CAD build for the part. Positions are in the model's coordinates, mm. A direction names the side the tool comes from. Coordinates: 2 decimals unless noted, no trailing zeros. Loops run counter-clockwise (first coordinate to the right, second up) from the corner with the lowest first, then second, coordinate; pieces in that order, holes last. Notation, with made-up numbers: (-6, 11.5) -> (53, 11.5) arc R25 cw to (53, 29.5) -> close; hole circle Ø1 at (3.25, 64). An arc over 180 degrees is marked (long way). Answer as CSV lines item,"result". Start each with the question number.
```python
from build123d import *

# Parameters (mm, degrees)
SKETCH1_W           = 152.4
SKETCH1_H           = 292.1
BOSS_EXTRUDE1_DEPTH = 3.048
SKETCH2_R           = 25.4
SKETCH2_R_2         = 10.7315
SKETCH2_R_3         = 2.0193
SKETCH2_W           = 16.173788568
SKETCH2_H           = 32.6898
CUT_EXTRUDE1_DEPTH  = 165.761442103
SKETCH4_W           = 55.88
SKETCH4_H           = 76.2
CUT_EXTRUDE2_DEPTH  = 165.761442103
SKETCH5_R           = 2.54
CUT_EXTRUDE3_DEPTH  = 165.761442103
SKETCH6_W           = 152.4
SKETCH6_H           = 5.08
CUT_EXTRUDE4_DEPTH  = 165.761442103
CUT_EXTRUDE5_DEPTH  = 6.35
FILLET1_R           = 6.35


with BuildPart() as part:
    # Sketch1 → Boss-Extrude1 (new body)
    with BuildSketch(Plane.XY):
        Rectangle(SKETCH1_W, SKETCH1_H)
    extrude(amount=BOSS_EXTRUDE1_DEPTH)

    # Sketch2 → Cut-Extrude1 (cut, through all)
    with BuildSketch(Plane.XY):
        with Locations(Location((0, -59.69, 0), (0, 0, 180))):
            Circle(SKETCH2_R)
        with Locations((0, 92.71)):
            Circle(SKETCH2_R_2)
        with Locations(Location((0, 38.1, 0), (0, 0, 180))):
            Circle(SKETCH2_R_3)
        with Locations(Location((0, 31.75, 0), (0, 0, 180))):
            Circle(SKETCH2_R_3)
        with Locations(Location((0, 25.4, 0), (0, 0, 180))):
            Circle(SKETCH2_R_3)
        with Locations(Location((0, 19.05, 0), (0, 0, 180))):
            Circle(SKETCH2_R_3)
        with Locations(Location((0, 12.7, 0), (0, 0, 180))):
            Circle(SKETCH2_R_3)
        with Locations(Location((0, 6.35, 0), (0, 0, 180))):
            Circle(SKETCH2_R_3)
        with Locations(Location((0, 0, 0), (0, 0, 180))):
            Circle(SKETCH2_R_3)
        with Locations(Location((0, -6.35, 0), (0, 0, 180))):
            Circle(SKETCH2_R_3)
        with Locations((0, 92.71)):
            Rectangle(SKETCH2_W, SKETCH2_H)
    extrude(amount=CUT_EXTRUDE1_DEPTH, mode=Mode.SUBTRACT)

    # Sketch4 → Cut-Extrude2 (cut, through all)
    with BuildSketch(Plane.XY):
        with Locations((48.26, 107.95)):
            Rectangle(SKETCH4_W, SKETCH4_H)
    extrude(amount=CUT_EXTRUDE2_DEPTH, mode=Mode.SUBTRACT)

    # Sketch5 → Cut-Extrude3 (cut, through all)
    with BuildSketch(Plane(origin=(0, 0, 0), x_dir=(-1, 0, 0), z_dir=(0, 0, -1))):
        with Locations((-38.1, -106.299)):
            Circle(SKETCH5_R)
        with Locations((-63.5, -106.299)):
            Circle(SKETCH5_R)
        with Locations((63.5, -106.299)):
            Circle(SKETCH5_R)
        with Locations((38.1, -106.299)):
            Circle(SKETCH5_R)
    extrude(amount=-CUT_EXTRUDE3_DEPTH, mode=Mode.SUBTRACT)

    # Sketch6 → Cut-Extrude4 (cut, through all)
    with BuildSketch(Plane(origin=(0, 0, 0), x_dir=(-1, 0, 0), z_dir=(0, 0, -1))):
        with Locations((0, -143.51)):
            Rectangle(SKETCH6_W, SKETCH6_H)
    extrude(amount=-CUT_EXTRUDE4_DEPTH, mode=Mode.SUBTRACT)

    # Sketch7 → Cut-Extrude5 (cut)
    with BuildSketch(Plane(origin=(0, 0, 0), x_dir=(-1, 0, 0), z_dir=(0, 0, -1))):
        with BuildLine():
            Line((63.5, 133.35), (15.671209909, 133.35))
            Line((15.671209909, 133.35), (15.671209909, -24.962155552))
            ThreePointArc((15.671209909, -24.962155552), (32.005336255, -39.019527068), (38.1, -59.69))
            Line((38.1, -59.69), (63.5, -59.69))
            Line((63.5, -59.69), (63.5, 133.35))
        make_face()
    extrude(amount=-CUT_EXTRUDE5_DEPTH, mode=Mode.SUBTRACT)

    # Fillet1
    fillet1_edges = [part.edges().sort_by_distance(p)[0] for p in [
        (-38.1, -59.69, 1.524),
        (-15.671209909, -24.962155552, 1.524),
        (-15.671209909, 133.35, 1.524),
        (-63.5, 133.35, 1.524),
        (-63.5, -59.69, 1.524),
    ]]
    fillet(fillet1_edges, radius=FILLET1_R)


solid = part.part
```
Q1. Saw through at A-A (x = 28). List the corners of the cut face in (y, z), and give its area (3 significant figures).
Q2. Saw through at B-B (z = 2.35). Give the number of separate pieces and of enclosed holes in the cut face, and give its area (3 significant figures).
Q3. Pin check, flat tips, straight feed: pin 1 Ø3.5 at (x, y) = (0, 19.05) entering from -Z; pin 2 Ø8 at (x, y) = (-38.1, -106.299) entering from -Z; pin 3 Ø1.5 at (x, z) = (60.5, 1.5) entering from +Y; pin 4 Ø1.5 at (y, z) = (105, 2) entering from +X. Stop position of each tip, or through.
Q4. Two-plate mould, pull along X, no slides. Class faces 1 (the flat face through (-1, -27, 0)), 2 (the cylindrical face through (-64.87, -104.16, 1.5)): pulls with the +X half, pulls with the -X half, needs draft (parallel to the pull), parting line crosses it, or undercut.
Q5. Probe probe 1 along X at (y, z) = (25.4, 1.55); probe 2 along Y at (x, z) = (63.5, 1.5); probe 3 along X at (y, z) = (-56.5, 1.1). List the from-to ranges inside material, lowest first. Write a range as from..to.
Q6. Which spindle directions (+Z, -Z, +X, -X, +Y, -Y) get a long thin tool onto all of the face, cutting with end or side? Do faces 3 (the cylindrical face through (-61.69, 131.44, 1.55)), 4 (the flat face through (-1, -27, 3.048)). Say none if no direction does.
Ans:
1,outline,"(-140.97, 0) -> (69.85, 0) -> (69.85, 3.05) -> (-140.97, 3.05) -> close"
1,area,"643 mm²"
2,separate pieces,"1"
2,enclosed holes,"15"
2,area,"28,100 mm²"
3,pin 1,"passes through"
3,pin 2,"stops at z = 0"
3,pin 3,"stops at y = 69.85"
3,pin 4,"stops at x = 20.32"
4,face 1,"needs draft"
4,face 2,"undercut"
5,probe 1,"x = -76.2..-63.5, -15.67..-2.02, 2.02..76.2"
5,probe 2,"y = -140.97..-108.84, -103.76..69.85"
5,probe 3,"x = -76.2..-62.66, -38.49..-25.2, 25.2..76.2"
6,face 3,"+Z, -Z"
6,face 4,"+Z, +X, -X, +Y, -Y"
